Geometry check sheet. Reference: drawing and pictorial views, mm from the part's lowest x, y, z. Give positions to 0.01 mm unless a question says otherwise; leave off trailing zeros. Order: outer loops, then holes, each group sorted by start corner. A loop starts at its lowest first (then second) coordinate and runs counter-clockwise, first axis right, second up. Notation, with made-up numbers: M -8,-17 L 14,-17 A15 cw 14,10 Z; hole C 54,18.5 d8. An arc over 180 degrees is marked long. Answer as a JSON object with one key per item and string values. Group by question number.
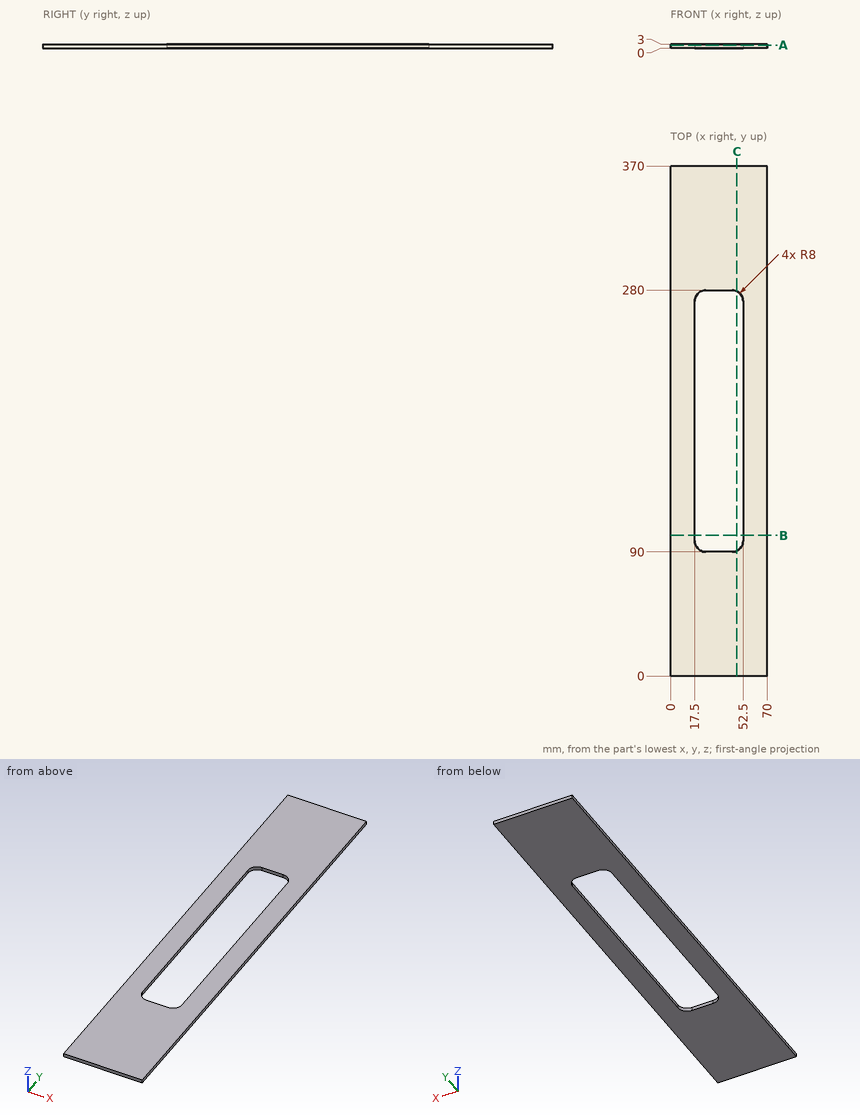
1. Cross-section at B-B (y = 102). Record the cut outline in (x, z).
2. Cross-section at C-C (x = 48). Record the cut outline in (y, z).
3. Cross-section at A-A (z = 2.1). Record the cut outline in (x, y).
4. Thickness scan on line 1 along Y through (x, z) = (34, 2.6); line 2 along X through (y, z) = (220, 1.5). Record the ranges inside material, lowest first. Write a range as [from, to].
Report:
{
 "1": {"outline": "M 0,0 L 17.5,0 L 17.5,3 L 0,3 Z; M 52.5,0 L 70,0 L 70,3 L 52.5,3 Z"},
 "2": {"outline": "M 0,0 L 90.81,0 L 90.81,3 L 0,3 Z; M 279.19,0 L 370,0 L 370,3 L 279.19,3 Z"},
 "3": {"outline": "M 0,0 L 70,0 L 70,370 L 0,370 Z; hole M 17.5,98 A8 ccw 25.5,90 L 44.5,90 A8 ccw 52.5,98 L 52.5,272 A8 ccw 44.5,280 L 25.5,280 A8 ccw 17.5,272 Z"},
 "4": {"line 1": "y = [0, 90], [280, 370]", "line 2": "x = [0, 17.5], [52.5, 70]"}
}
